```python
from build123d import *

# Parameters (mm, degrees)
SKETCH2_R                      = 27.42
BOSS_EXTRUDE1_DEPTH            = 12
CUT_EXTRUDE1_DEPTH             = 13
SKETCH3_R                      = 2.085
CUT_EXTRUDE2_DEPTH             = 13
CIRPATTERN1_COUNT              = 4
CUT_EXTRUDE4_DEPTH             = 13
CIRPATTERN2_COUNT              = 4
F_6_0_204_DIAMETER_HOLE1_D     = 5.1816
F_6_0_204_DIAMETER_HOLE1_DEPTH = 12
F_6_0_204_DIAMETER_HOLE1_TIP   = 1.556709692
CUT_EXTRUDE5_DEPTH             = 3.08


with BuildPart() as part:
    # Sketch2 → Boss-Extrude1 (new body)
    with BuildSketch(Plane(origin=(0, 0, 0), x_dir=(1, 0, 0), z_dir=(0, 1, 0))):
        Circle(SKETCH2_R)
    extrude(amount=BOSS_EXTRUDE1_DEPTH)

    # Sketch1 → Cut-Extrude1 (cut, through all)
    with BuildSketch(Plane(origin=(0, 0, 0), x_dir=(1, 0, 0), z_dir=(0, 1, 0))):
        with BuildLine():
            Line((0, 21.9), (0, 27.42))
            ThreePointArc((0, 27.42), (-10.493179715, 25.332776781), (-19.38886794, 19.38886794))
            Line((-19.38886794, 19.38886794), (-15.485638508, 15.485638508))
            ThreePointArc((-15.485638508, 15.485638508), (-8.380767169, 20.232961762), (0, 21.9))
        make_face()
        with BuildLine():
            Line((0, -21.9), (0, -27.42))
            ThreePointArc((0, -27.42), (10.493179715, -25.332776781), (19.38886794, -19.38886794))
            Line((19.38886794, -19.38886794), (15.485638508, -15.485638508))
            ThreePointArc((15.485638508, -15.485638508), (8.380767169, -20.232961762), (0, -21.9))
        make_face()
        with BuildLine():
            Line((21.9, 0), (27.42, 0))
            ThreePointArc((27.42, 0), (25.332776781, 10.493179715), (19.38886794, 19.38886794))
            Line((19.38886794, 19.38886794), (15.485638508, 15.485638508))
            ThreePointArc((15.485638508, 15.485638508), (20.232961762, 8.380767169), (21.9, 0))
        make_face()
        with BuildLine():
            Line((-21.9, 0), (-27.42, 0))
            ThreePointArc((-27.42, 0), (-25.332776781, -10.493179715), (-19.38886794, -19.38886794))
            Line((-19.38886794, -19.38886794), (-15.485638508, -15.485638508))
            ThreePointArc((-15.485638508, -15.485638508), (-20.232961762, -8.380767169), (-21.9, 0))
        make_face()
    extrude(amount=CUT_EXTRUDE1_DEPTH, mode=Mode.SUBTRACT)

    # Sketch3 → Cut-Extrude2 (cut, through all)
    with BuildSketch(Plane(origin=(0, 12, 0), x_dir=(1, 0, 0), z_dir=(0, 1, 0))):
        with Locations((12.77, 0)):
            Circle(SKETCH3_R)
    cut_extrude2 = extrude(amount=-CUT_EXTRUDE2_DEPTH, mode=Mode.SUBTRACT)

    # CirPattern1: Cut-Extrude2 ×4 about axis
    cirpattern1_axis = Axis((0, 0, 0), (0, 1, 0))
    for i in range(1, CIRPATTERN1_COUNT):
        add(cut_extrude2.rotate(cirpattern1_axis, i * 360 / CIRPATTERN1_COUNT), mode=Mode.SUBTRACT)

    # Sketch5 → Cut-Extrude4 (cut, through all)
    with BuildSketch(Plane(origin=(0, 12, 0), x_dir=(1, 0, 0), z_dir=(0, 1, 0))):
        Polygon((-5.464214141, 17.11146878), (-7.413599954, 21.81770245), (-10.185238552, 20.669652153), (-8.235852738, 15.963418483), (-6.850033439, 16.537443632), align=None)
    cut_extrude4 = extrude(amount=-CUT_EXTRUDE4_DEPTH, mode=Mode.SUBTRACT)

    # CirPattern2: Cut-Extrude4 ×4 about axis
    cirpattern2_axis = Axis((0, 0, 0), (0, 1, 0))
    for i in range(1, CIRPATTERN2_COUNT):
        add(cut_extrude4.rotate(cirpattern2_axis, i * 360 / CIRPATTERN2_COUNT), mode=Mode.SUBTRACT)

    # #6 (0.204) Diameter Hole1
    with Locations(Plane(origin=(0, 12, 0), x_dir=(1, 0, 0), z_dir=(0, 1, 0))):
        with Locations((0, 0)):
            Hole(F_6_0_204_DIAMETER_HOLE1_D / 2, depth=F_6_0_204_DIAMETER_HOLE1_DEPTH)
            with Locations((0, 0, -(F_6_0_204_DIAMETER_HOLE1_DEPTH + F_6_0_204_DIAMETER_HOLE1_TIP / 2))):  # 118° drill point
                Cone(0, F_6_0_204_DIAMETER_HOLE1_D / 2, F_6_0_204_DIAMETER_HOLE1_TIP, mode=Mode.SUBTRACT)

    # Sketch8 → Cut-Extrude5 (cut)
    with BuildSketch(Plane(origin=(0, 12, 0), x_dir=(1, 0, 0), z_dir=(0, 1, 0))):
        Polygon((2.453738644, -4.25), (4.907477288, 0), (2.453738644, 4.25), (-2.453738644, 4.25), (-4.907477288, 0), (-2.453738644, -4.25), align=None)
    extrude(amount=-CUT_EXTRUDE5_DEPTH, mode=Mode.SUBTRACT)


solid = part.part
```
Geometry check sheet. Reference: the model listing, model coordinates, mm. A direction names the side the tool comes from. Coordinates: 2 decimals unless noted, no trailing zeros. Loops run counter-clockwise (first coordinate to the right, second up) from the corner with the lowest first, then second, coordinate; pieces in that order, holes last. Notation, with made-up numbers: (40, 43.5) -> (69, 43.5) arc R30 ccw to (69, 75.5) -> close; hole circle Ø3 at (25, 23.5). An arc over 180 degrees is marked (long way). Put each result on its own line as item: value.
1) Cross-section at B-B on z = 12.77. Record the boundary of the cut face in (x, y) (3 decimals).
Result set:
outline: (-17.791, 0) -> (-2.085, 0) -> (-2.085, 12) -> (-17.791, 12) -> close; (2.085, 0) -> (24.265, 0) -> (24.265, 12) -> (2.085, 12) -> close
2) Gauge pin test, flat ends, axial feed: pin 1 Ø5 at (y, z) = (8, -12) entering from -X; pin 2 Ø1 at (y, z) = (5, 9.5) entering from -X; pin 3 Ø1 at (x, y) = (-15.5, 6) entering from +Z. Record the tip position at first contact, or that the pin passes through.
Result set:
pin 1: stops at x = -25.72
pin 2: stops at x = -19.61
pin 3: stops at z = 22.95
3) Release check for a two-part mould opening along X. For faces 6 (the cylindrical face through (-21.605, 5.916, 3.583)), 7 (the cylindrical face through (10.632, 5.916, -25.275)), 8 (the flat face through (-3.698, 10.482, 2.095)) record: released by +X, released by -X, zero draft, split by the parting line, or undercut.
Result set:
face 6: released by -X
face 7: released by +X
face 8: undercut
4) Thickness scan on line 1 (X direction, y = 2.25, z = -19); line 2 (Z direction, x = -18.5, y = 9.75); line 3 (X direction, y = 2, z = 6). Record the ranges inside material, lowest first.
Result set:
line 1: x = -19.77 to -19, -10.89 to -9.49, -6.25 to 19
line 2: z = -18.5 to 6.04, 9.29 to 11.72, 18.5 to 20.24
line 3: x = -21.06 to -18.4, -16.89 to 26.76
5) Cross-section at A-A on x = 12.77. Record the boundary of the cut face in (y, z) (3 decimals), plus the area to 3 significant figures.
Result set:
outline: (0, -24.265) -> (12, -24.265) -> (12, -2.085) -> (0, -2.085) -> close; (0, 2.085) -> (12, 2.085) -> (12, 17.791) -> (0, 17.791) -> close
area: 455 mm^2
6) Tool access check on faces 1 (the flat face through (0, 10, -4.25)), 2 (the cylindrical face through (-17.753, 5.916, 12.824)), 3 (the flat face through (9, 6.08, 17.81)), 4 (the flat face through (-25, 6, 0)), 5 (the flat face through (-18.91, 6.08, 6.21)). Record the directions out of +Z, -Z, +X, -X, +Y, -Y that give a thin tool (end or side, any length) a straight path to the whole face; none if there is none.
Result set:
face 1: +Y
face 2: -X, +Y, -Y
face 3: +Z, +Y, -Y
face 4: +Z, -X, +Y, -Y
face 5: +Y, -Y
7) Cross-section at D-D on x = -24. Record the boundary of the cut face in (y, z), plus the area to 3 significant figures.
Result set:
outline: (0, -13.26) -> (12, -13.26) -> (12, 0) -> (0, 0) -> close
area: 159 mm^2
8) Cross-section at C-C on y = 11.25. Count the separate pieces of the cut face and the enclosed holes in it, plus the area to 3 significant figures.
Result set:
separate pieces: 1
enclosed holes: 5
area: 1,770 mm^2
